from build123d import *

# Parameters (mm, degrees)
SKETCH1_W                    = 100
SKETCH1_H                    = 100
BOSS_EXTRUDE1_DEPTH          = 30
SKETCH2_W                    = 95
SKETCH2_H                    = 95
CUT_EXTRUDE1_DEPTH           = 2.25
SKETCH3_W                    = 88
SKETCH3_H                    = 88
BOSS_EXTRUDE2_DEPTH          = 2.25
SKETCH4_W                    = 80
SKETCH4_H                    = 80
CUT_EXTRUDE2_DEPTH           = 15
F_9_16_CLEARANCE_HOLE1_D     = 14.7
F_5_16_CLEARANCE_HOLE1_D     = 8.7
F_5_16_CLEARANCE_HOLE1_DEPTH = 30
FILLET1_R                    = 5
FILLET2_R                    = 12
FILLET3_R                    = 15.5


with BuildPart() as part:
    # Sketch1 → Boss-Extrude1 (new body)
    with BuildSketch(Plane.XY.offset(30)):
        with Locations((49.999998297, 50.00000012)):
            Rectangle(SKETCH1_W, SKETCH1_H)
    extrude(amount=-BOSS_EXTRUDE1_DEPTH)

    # Sketch2 → Cut-Extrude1 (cut)
    with BuildSketch(Plane.XY.offset(30)):
        with Locations((49.999998297, 50.00000012)):
            Rectangle(SKETCH2_W, SKETCH2_H)
    extrude(amount=-CUT_EXTRUDE1_DEPTH, mode=Mode.SUBTRACT)

    # Sketch3 → Boss-Extrude2 (add)
    with BuildSketch(Plane.XY.offset(27.75)):
        with Locations((49.999998297, 50.00000012)):
            Rectangle(SKETCH3_W, SKETCH3_H)
    extrude(amount=BOSS_EXTRUDE2_DEPTH)

    # Sketch4 → Cut-Extrude2 (cut)
    with BuildSketch(Plane.XY.offset(30)):
        with Locations((49.999998297, 50.00000012)):
            Rectangle(SKETCH4_W, SKETCH4_H)
    extrude(amount=-CUT_EXTRUDE2_DEPTH, mode=Mode.SUBTRACT)

    # 9/16 Clearance Hole1 (through all)
    with Locations(Plane.XY.offset(15)):
        with Locations((50.000229381, 49.999170193)):
            Hole(F_9_16_CLEARANCE_HOLE1_D / 2)

    # 5/16 Clearance Hole1
    with Locations(Plane(origin=(0, 0, 0), x_dir=(-1, 0, 0), z_dir=(0, 0, -1))):
        with Locations((-79.999998297, 20.00000012)):
            Hole(F_5_16_CLEARANCE_HOLE1_D / 2, depth=F_5_16_CLEARANCE_HOLE1_DEPTH)

    # Fillet1
    fillet1_edges = [part.edges().sort_by_distance(p)[0] for p in [
        (9.999998297, 90.00000012, 22.5),
        (89.999998297, 90.00000012, 22.5),
        (89.999998297, 10.00000012, 22.5),
        (9.999998297, 10.00000012, 22.5),
        (57.350229381, 49.999170193, 15),
        (-1.703e-06, 1.2e-07, 15),
        (-1.703e-06, 100.00000012, 15),
        (99.999998297, 100.00000012, 15),
        (99.999998297, 1.2e-07, 15),
    ]]
    fillet(fillet1_edges, radius=FILLET1_R)

    # Fillet2
    fillet2_edges = [part.edges().sort_by_distance(p)[0] for p in [
        (5.999998297, 6.00000012, 28.875),
        (93.999998297, 6.00000012, 28.875),
        (93.999998297, 94.00000012, 28.875),
        (5.999998297, 94.00000012, 28.875),
    ]]
    fillet(fillet2_edges, radius=FILLET2_R)

    # Fillet3
    fillet3_edges = [part.edges().sort_by_distance(p)[0] for p in [
        (2.499998297, 2.50000012, 28.875),
        (2.499998297, 97.50000012, 28.875),
        (97.499998297, 97.50000012, 28.875),
        (97.499998297, 2.50000012, 28.875),
    ]]
    fillet(fillet3_edges, radius=FILLET3_R)


solid = part.part
Source: CAD feature listing. Evaluate the final solid. Frame: model axes, mm. A direction names the side the tool comes from. Coordinates: 2 decimals unless noted, no trailing zeros. Order: outer loops, then holes, each group sorted by start corner. A loop starts at its lowest first (then second) coordinate and runs counter-clockwise, first axis right, second up. Notation, with made-up numbers: M 14.25,-16.75 L 21.25,-16.75 A28 cw 21.25,9.25 Z; hole C 51.5,72.25 d3. An arc over 180 degrees is marked long. Write each question's results on one line, items separated by ' | '. Start each with the question number.
Item 1: Cut plane A-A (y = 20). Return loops of the section in (x, z), and give its area (3 significant figures).
Item 2: First-contact query: pin 1 Ø2 at (x, y) = (87, 35.5) entering from +Z; pin 2 Ø2 at (x, y) = (55, 85.5) entering from -Z. Flat tips, straight axial feed; report the tip coordinate or a pass-through.
Item 3: Set-up query: faces 4 (the face through (84.15, 21.31, 7.61)), 5 (the face through (90.58, 90.39, 28.89)). Return all of +Z, -Z, +X, -X, +Y, -Y with unobstructed straight access to the full face (end or side cutting, diameter ignored); none if empty.
Item 4: Cut plane B-B (z = 23.75). Return loops of the section in (x, y).
Item 5: Cut plane D-D (z = 13.5). Return loops of the section in (x, y).
Item 6: Line query: probe 1 along Y at (x, z) = (59, 28); probe 2 along Y at (x, z) = (51, 20.5). Output: solid intervals per line, ascending.
Item 7: Draft query along X for faces 1 (the face through (98, 1, 15)), 2 (the face through (6.92, 7.16, 28.86)), 3 (the face through (38, 51, 0)). Return one class per face: pulls with the +X half, pulls with the -X half, needs draft (parallel to the pull), parting line crosses it, or undercut.
Item 8: Cut plane C-C (x = 64.5). Return loops of the section in (y, z), and give its area (3 significant figures).
Checked values:
1) outline: M 0,0 L 75.65,0 L 75.65,15 L 10,15 L 10,30 L 6,30 L 6,27.75 L 2.5,27.75 L 2.5,30 L 0,30 Z; M 84.35,0 L 100,0 L 100,30 L 97.5,30 L 97.5,27.75 L 94,27.75 L 94,30 L 90,30 L 90,15 L 84.35,15 Z | area: 1,650 mm2
2) pin 1: stops at z = 15 | pin 2: stops at z = 0
3) face 4: +Z, -Z | face 5: +Z
4) outline: M 0,5 A5 ccw 5,0 L 95,0 A5 ccw 100,5 L 100,95 A5 ccw 95,100 L 5,100 A5 ccw 0,95 Z; hole M 10,15 A5 ccw 15,10 L 85,10 A5 ccw 90,15 L 90,85 A5 ccw 85,90 L 15,90 A5 ccw 10,85 Z
5) outline: M 0,5 A5 ccw 5,0 L 95,0 A5 ccw 100,5 L 100,95 A5 ccw 95,100 L 5,100 A5 ccw 0,95 Z; hole C 50,50 d17.56; hole C 80,20 d8.7
6) probe 1: y = 0 to 2.5, 6 to 10, 90 to 94, 97.5 to 100 | probe 2: y = 0 to 10, 90 to 100
7) face 1: pulls with the +X half | face 2: undercut | face 3: needs draft
8) outline: M 0,0 L 100,0 L 100,30 L 97.5,30 L 97.5,27.75 L 94,27.75 L 94,30 L 90,30 L 90,15 L 10,15 L 10,30 L 6,30 L 6,27.75 L 2.5,27.75 L 2.5,30 L 0,30 Z | area: 1,780 mm2
